Build history of the part. All positions in model axes, mm. Give positions to 0.01 mm unless a question says otherwise; leave off trailing zeros. Loops run counter-clockwise (first coordinate to the right, second up) from the corner with the lowest first, then second, coordinate; pieces in that order, holes last. Notation, with made-up numbers: (65.5, 14.25) - (114.5, 14.25) arc R28 ccw to (114.5, 51.25) - close; hole circle Ø2 at (12.5, 54). An arc over 180 degrees is marked (long way). Return JSON: item names as keys, results as strings. Group by question number.
1) Slice it at A-A (x = 25.5). List the corners of the cut face in (y, z), and give its area (3 significant figures).
2) Slice it at B-B (y = -42). List the corners of the cut face in (x, z).
3) Drop a flat-ended pin along its axis: pin 1 (2.5 mm diameter, centred on x = -41.04, y = -21, fed in from +Z). Give the stop position or say it passes through.
4) Slice it at C-C (z = 2.9). Count the separate pieces of the cut face and the enclosed holes in it, and give its area (3 significant figures).
5) Drill centre lines: probe 1 along X at (y, z) = (122, 4.65); probe 2 along Y at (x, z) = (28.5, 3.6); probe 3 along X at (y, z) = (1.5, 1.4). Where is each one in solid material? Low to high. Write a range as from..to.
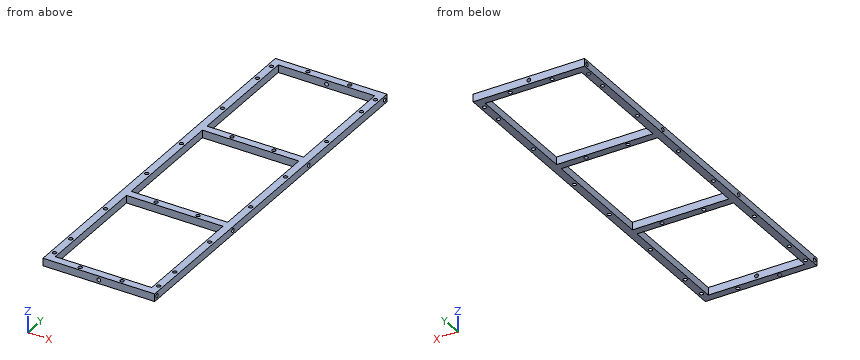
```python
from build123d import *

# Parameters (mm, degrees)
SKETCH1_W           = 88
SKETCH1_H           = 300
SKETCH1_W_2         = 76
SKETCH1_H_2         = 92
BOSS_EXTRUDE1_DEPTH = 6
SKETCH2_R           = 1.5
CUT_EXTRUDE1_DEPTH  = 10
SKETCH3_R           = 1.5
CUT_EXTRUDE2_DEPTH  = 10
SKETCH4_R           = 1.5
CUT_EXTRUDE3_DEPTH  = 10
SKETCH5_R           = 1.5
CUT_EXTRUDE4_DEPTH  = 10


with BuildPart() as part:
    # Sketch1 → Boss-Extrude1 (new body)
    with BuildSketch(Plane.XY):
        Rectangle(SKETCH1_W, SKETCH1_H)
        with Locations((0, 98)):
            Rectangle(SKETCH1_W_2, SKETCH1_H_2, mode=Mode.SUBTRACT)
        with Locations((0, -98)):
            Rectangle(SKETCH1_W_2, SKETCH1_H_2, mode=Mode.SUBTRACT)
        Rectangle(SKETCH1_W_2, SKETCH1_H_2, mode=Mode.SUBTRACT)
    extrude(amount=BOSS_EXTRUDE1_DEPTH)

    # Sketch2 → Cut-Extrude1 (cut)
    with BuildSketch(Plane(origin=(44, 0, 0), x_dir=(0, 0, -1), z_dir=(1, 0, 0))):
        with Locations((-3, 147)):
            Circle(SKETCH2_R)
        with Locations((-3, 49)):
            Circle(SKETCH2_R)
        with Locations((-3, -49)):
            Circle(SKETCH2_R)
        with Locations((-3, -147)):
            Circle(SKETCH2_R)
    cut_extrude1 = extrude(amount=-CUT_EXTRUDE1_DEPTH, mode=Mode.SUBTRACT)

    # Mirror1: Cut-Extrude1 across plane
    add(cut_extrude1.mirror(Plane(origin=(0, 0, 0), x_dir=(0, 0, 1), z_dir=(1, 0, 0))), mode=Mode.SUBTRACT)

    # Sketch3 → Cut-Extrude2 (cut)
    with BuildSketch(Plane.XY.offset(6)):
        with Locations((-41, 140)):
            Circle(SKETCH3_R)
        with Locations((41, 140)):
            Circle(SKETCH3_R)
        with Locations((41, -140)):
            Circle(SKETCH3_R)
        with Locations((-41, -140)):
            Circle(SKETCH3_R)
    extrude(amount=-CUT_EXTRUDE2_DEPTH, mode=Mode.SUBTRACT)

    # Sketch4 → Cut-Extrude3 (cut)
    with BuildSketch(Plane.XY.offset(6)):
        with Locations((-16.5, 147)):
            Circle(SKETCH4_R)
        with Locations((16.5, 147)):
            Circle(SKETCH4_R)
        with Locations((16.5, 49)):
            Circle(SKETCH4_R)
        with Locations((-16.5, 49)):
            Circle(SKETCH4_R)
        with Locations((16.5, -49)):
            Circle(SKETCH4_R)
        with Locations((-16.5, -49)):
            Circle(SKETCH4_R)
        with Locations((16.5, -147)):
            Circle(SKETCH4_R)
        with Locations((-16.5, -147)):
            Circle(SKETCH4_R)
        with Locations((-41.040928423, 122)):
            Circle(SKETCH4_R)
        with Locations((-41.040928423, 77)):
            Circle(SKETCH4_R)
        with Locations((40.959071577, 122)):
            Circle(SKETCH4_R)
        with Locations((40.959071577, 77)):
            Circle(SKETCH4_R)
        with Locations((40.959071577, 24)):
            Circle(SKETCH4_R)
        with Locations((40.959071577, -21)):
            Circle(SKETCH4_R)
        with Locations((40.959071577, -74)):
            Circle(SKETCH4_R)
        with Locations((40.959071577, -119)):
            Circle(SKETCH4_R)
        with Locations((-41.040928423, 24)):
            Circle(SKETCH4_R)
        with Locations((-41.040928423, -21)):
            Circle(SKETCH4_R)
        with Locations((-41.040928423, -74)):
            Circle(SKETCH4_R)
        with Locations((-41.040928423, -119)):
            Circle(SKETCH4_R)
    extrude(amount=-CUT_EXTRUDE3_DEPTH, mode=Mode.SUBTRACT)

    # Sketch5 → Cut-Extrude4 (cut)
    with BuildSketch(Plane(origin=(0, 150, 0), x_dir=(1, 0, 0), z_dir=(0, 1, 0))):
        with Locations(Location((0, -3, 0), (0, 0, 270))):
            Circle(SKETCH5_R)
    cut_extrude4 = extrude(amount=-CUT_EXTRUDE4_DEPTH, mode=Mode.SUBTRACT)

    # Mirror2: Cut-Extrude4 across plane
    add(cut_extrude4.mirror(Plane.ZX), mode=Mode.SUBTRACT)


solid = part.part
```
Results:
{
 "1": {"outline": "(-150, 0) - (-144, 0) - (-144, 6) - (-150, 6) - close; (-52, 0) - (-46, 0) - (-46, 6) - (-52, 6) - close; (46, 0) - (52, 0) - (52, 6) - (46, 6) - close; (144, 0) - (150, 0) - (150, 6) - (144, 6) - close", "area": "144 mm2"},
 "2": {"outline": "(-44, 0) - (-38, 0) - (-38, 6) - (-44, 6) - close; (38, 0) - (44, 0) - (44, 6) - (38, 6) - close"},
 "3": {"pin 1": "through"},
 "4": {"separate pieces": "1", "enclosed holes": "25", "area": "4,980 mm2"},
 "5": {"probe 1": "-44..-42.54, -39.54..-38, 38..39.46, 42.46..44", "probe 2": "-150..-144, -52..-46, 46..52, 144..150", "probe 3": "-44..-38, 38..44"}
}
